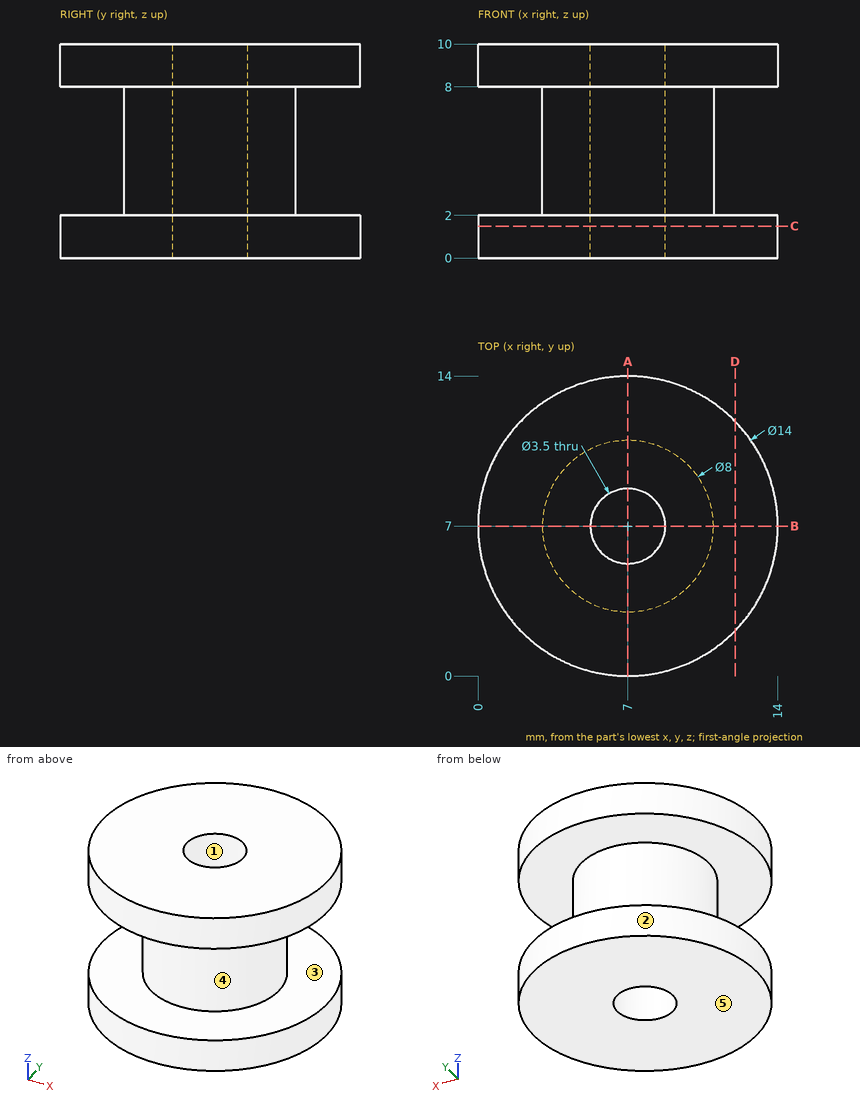
Can you work these out from the drawing? Everything is in mm from the part's minimum corner. A direction names the side the tool comes from. Coordinates: 2 decimals unless noted, no trailing zeros. Loops run counter-clockwise (first coordinate to the right, second up) from the corner with the lowest first, then second, coordinate; pieces in that order, holes last. Notation, with made-up numbers: (76, 0) - (101, 0) arc R27 ccw to (101, 35) - close; hole circle Ø9 at (21, 64). An arc over 180 degrees is marked (long way). Put each result on its own line as item: value. Start each with the question number.
Item 1: For pin 1 (1 mm diameter, centred on x = 4, z = 8, fed in from -Y); pin 2 (3 mm diameter, centred on x = 7, y = 7, fed in from +Z); pin 3 (1.5 mm diameter, centred on x = 9, z = 9, fed in from +Y); pin 4 (1 mm diameter, centred on y = 8, z = 5.5, fed in from -X), each with a flat end and sliding along its axis, tell me the tip position at first contact or that it passes through.
Item 2: Which directions (+Z, -Z, +X, -X, +Y, -Y) give clear straight access to the entire face, cutting with the end or side of a thin tool? Please do the marked faces 4 and 5.
Item 3: Suppose I cut it at A-A (x = 7). Please give me the cut outline in (y, z).
Item 4: Suppose I cut it at C-C (z = 1.5). Please give me the cut outline in (x, y).
Item 5: If we mould it in two halves opening along Y, with no side actions, what happens to the marked faces 1, 2 and 3? For each: +Y half, -Y half, draft (parallel to the pull), parting line (faces both ways), or undercut.
Item 6: If I drill on line 1 along Z through (x, y) = (3.25, 5.5); line 2 along Y through (x, z) = (7, 6.25); line 3 along Y through (x, z) = (7, 9.25), over which ranges is the centre line in solid material (lowest first)?
Item 7: Suppose I cut it at D-D (x = 12). Please give me the cut outline in (y, z).
Here are the results:
1. pin 1: y = 0.46
1. pin 2: through
1. pin 3: y = 13.89
1. pin 4: x = 3.03
2. face 4: none
2. face 5: -Z, +X, -X, +Y, -Y
3. outline: (0, 0) - (5.25, 0) - (5.25, 10) - (0, 10) - (0, 8) - (3, 8) - (3, 2) - (0, 2) - close; (8.75, 0) - (14, 0) - (14, 2) - (11, 2) - (11, 8) - (14, 8) - (14, 10) - (8.75, 10) - close
4. outline: circle Ø14 at (7, 7); hole circle Ø3.5 at (7, 7)
5. face 1: undercut
5. face 2: parting line
5. face 3: draft
6. line 1: 0 to 2, 8 to 10
6. line 2: 3 to 5.25, 8.75 to 11
6. line 3: 0 to 5.25, 8.75 to 14
7. outline: (2.1, 0) - (11.9, 0) - (11.9, 2) - (2.1, 2) - close; (2.1, 8) - (11.9, 8) - (11.9, 10) - (2.1, 10) - close
